Geometry: see drawing. Coordinates: mm, zero at the bounding-box minimum. Round coordinates to 2 decimals unless told otherwise and drop trailing zeros. Loops run counter-clockwise (first coordinate to the right, second up) from the corner with the lowest first, then second, coordinate; pieces in that order, holes last. Notation, with made-up numbers: (64, -20.75) -> (116, -20.75) arc R17 ccw to (116, -0.75) -> close; hole circle Ø7 at (50.25, 50). An arc over 180 degrees is marked (long way). Write item = value, one per line.
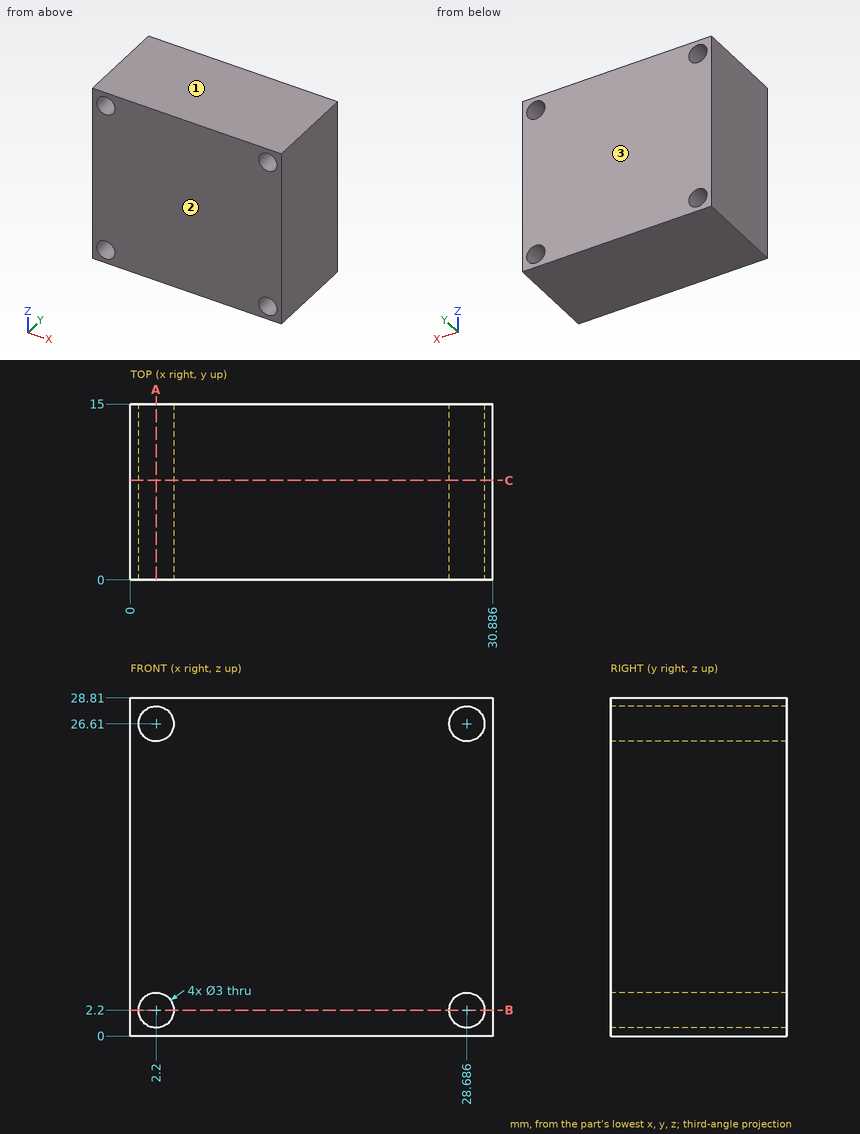
1. Section query C-C (y = 8.5). Return the cut outline in (x, z).
Evaluation:
outline = (0, 0) -> (30.89, 0) -> (30.89, 28.81) -> (0, 28.81) -> close; hole circle Ø3 at (2.2, 2.2); hole circle Ø3 at (2.2, 26.61); hole circle Ø3 at (28.69, 2.2); hole circle Ø3 at (28.69, 26.61)
2. Section query B-B (z = 2.2). Return the cut outline in (x, y).
Evaluation:
outline = (0, 0) -> (0.7, 0) -> (0.7, 15) -> (0, 15) -> close; (3.7, 0) -> (27.19, 0) -> (27.19, 15) -> (3.7, 15) -> close; (30.19, 0) -> (30.89, 0) -> (30.89, 15) -> (30.19, 15) -> close
3. Mould query, pull axis Y, two halves, no side actions, for the marked faces 1, 2 and 3. Classes: released by +Y, released by -Y, zero draft, split by the parting line, or undercut.
Evaluation:
face_1 = zero draft
face_2 = released by -Y
face_3 = released by +Y
4. Section query A-A (x = 2.2). Return the cut outline in (y, z).
Evaluation:
outline = (0, 0) -> (15, 0) -> (15, 0.7) -> (0, 0.7) -> close; (0, 3.7) -> (15, 3.7) -> (15, 25.11) -> (0, 25.11) -> close; (0, 28.11) -> (15, 28.11) -> (15, 28.81) -> (0, 28.81) -> close
5. Line query: probe 1 along Z at (x, y) = (2.2, 3.5); probe 2 along X at (y, z) = (2, 26) (1 decimal); probe 3 along X at (y, z) = (7, 27.25) (1 decimal). Output: solid intervals per line, ascending. Write a range as from..to.
Evaluation:
probe_1 = 0..0.7, 3.7..25.11, 28.11..28.81
probe_2 = 0..0.8, 3.6..27.3, 30.1..30.9
probe_3 = 0..0.8, 3.6..27.3, 30..30.9
